from build123d import *

# Parameters (mm, degrees)
SKETCH_1_W          = 38
SKETCH_1_H          = 30
EXTRUDE_1_DEPTH     = 3
SKETCH_2_R          = 1.55
CUT_EXTRUDE_1_DEPTH = 10
SKETCH_3_W          = 22
SKETCH_3_H          = 22.358896132
CUT_EXTRUDE_2_DEPTH = 10
FILLET_1_R          = 7
FILLET_2_R          = 7
FILLET_3_R          = 3


with BuildPart() as part:
    # 草图1 → 凸台-拉伸1 (new body)
    with BuildSketch(Plane.XY):
        Rectangle(SKETCH_1_W, SKETCH_1_H)
    extrude(amount=EXTRUDE_1_DEPTH)

    # 草图2 → 切除-拉伸1 (cut)
    with BuildSketch(Plane.XY.offset(3)):
        with Locations((0, 12)):
            Circle(SKETCH_2_R)
        with Locations((-15, -12)):
            Circle(SKETCH_2_R)
        with Locations((15, -12)):
            Circle(SKETCH_2_R)
        with BuildLine():
            Line((6.963744532, 13.55), (13.036255468, 13.55))
            ThreePointArc((13.036255468, 13.55), (14.586255468, 12), (13.036255468, 10.45))
            Line((13.036255468, 10.45), (6.963744532, 10.45))
            ThreePointArc((6.963744532, 10.45), (5.413744532, 12), (6.963744532, 13.55))
        make_face()
        with BuildLine():
            Line((-6.963744532, 13.55), (-13.036255468, 13.55))
            ThreePointArc((-13.036255468, 13.55), (-14.586255468, 12), (-13.036255468, 10.45))
            Line((-13.036255468, 10.45), (-6.963744532, 10.45))
            ThreePointArc((-6.963744532, 10.45), (-5.413744532, 12), (-6.963744532, 13.55))
        make_face()
    extrude(amount=-CUT_EXTRUDE_1_DEPTH, mode=Mode.SUBTRACT)

    # 草图3 → 切除-拉伸2 (cut)
    with BuildSketch(Plane.XY.offset(3)):
        with Locations((0, -3.820551934)):
            Rectangle(SKETCH_3_W, SKETCH_3_H)
    extrude(amount=-CUT_EXTRUDE_2_DEPTH, mode=Mode.SUBTRACT)

    # 圆角1
    fillet_1_edges = [part.edges().sort_by_distance(p)[0] for p in [
        (-19, 15, 1.5),
        (19, 15, 1.5),
    ]]
    fillet(fillet_1_edges, radius=FILLET_1_R)

    # 圆角2
    fillet_2_edges = [part.edges().sort_by_distance(p)[0] for p in [
        (11, 7.358896132, 1.5),
        (-11, 7.358896132, 1.5),
    ]]
    fillet(fillet_2_edges, radius=FILLET_2_R)

    # 圆角3
    fillet_3_edges = [part.edges().sort_by_distance(p)[0] for p in [
        (11, -15, 1.5),
        (-11, -15, 1.5),
        (19, -15, 1.5),
        (-19, -15, 1.5),
    ]]
    fillet(fillet_3_edges, radius=FILLET_3_R)


solid = part.part
Geometry check sheet. Reference: the model listing, model coordinates, mm. A direction names the side the tool comes from. Round coordinates to 2 decimals unless told otherwise and drop trailing zeros. Order: outer loops, then holes, each group sorted by start corner. A loop starts at its lowest first (then second) coordinate and runs counter-clockwise, first axis right, second up. Notation, with made-up numbers: M -14,39.25 L 37,39.25 A29 cw 37,60.25 Z; hole C 55,77 d11. An arc over 180 degrees is marked long. Write each question's results on one line, items separated by ' | '. Start each with the question number.
1. Cross-section at B-B on z = 2.1. Record the boundary of the cut face in (x, y), plus the area to 3 significant figures.
2. Cross-section at A-A on x = 0. Record the boundary of the cut face in (y, z), plus the area to 3 significant figures.
3. Cross-section at C-C on y = -8.5. Record the boundary of the cut face in (x, z).
4. Go/stop test with flat-tipped pins: P1, Ø5, axis at x = -6, y = 0.5, coming from the -Z side; P2, Ø0.9, axis at x = -9.5, z = 2, coming from the -Y side. Record where each tip stops, or that it passes through.
5. Draft check along Y on faces 1 (the face through (-0.336, 10.487, 1.521)), 2 (the face through (0, 10, 3)), 3 (the face through (8.9, 5.36, 1.48)). Enter one of: pulls with the +Y half, pulls with the -Y half, needs draft (parallel to the pull), parting line crosses it, or undercut.
6. Set-up check for faces 4 (the face through (11, -6, 2)), 5 (the face through (10, 13.55, 2)), 6 (the face through (-15, -15, 1)): record each of +Z, -Z, +X, -X, +Y, -Y from which the full face is reachable in a straight line by a thin tool's end or side.
7. Cross-section at D-D on y = 12. Record the boundary of the cut face in (x, z), plus the area to 3 significant figures.
8. Material ranges on L1, parallel to X at y = 11.25, z = 2.55; L2, parallel to Y at x = 0, z = 1.75; L3, parallel to X at y = -11.25, z = 1.95, recorded low to high. Write a range as from..to.
Resolved:
1) outline: M -19,-12 A3 ccw -16,-15 L -14,-15 A3 ccw -11,-12 L -11,0.36 A7 cw -4,7.36 L 4,7.36 A7 cw 11,0.36 L 11,-12 A3 ccw 14,-15 L 16,-15 A3 ccw 19,-12 L 19,8 A7 ccw 12,15 L -12,15 A7 ccw -19,8 Z; hole C -15,-12 d3.1; hole M -13.04,10.45 L -6.96,10.45 A1.55 ccw -6.96,13.55 L -13.04,13.55 A1.55 ccw Z; hole C 0,12 d3.1; hole M 6.96,10.45 L 13.04,10.45 A1.55 ccw 13.04,13.55 L 6.96,13.55 A1.55 ccw Z; hole C 15,-12 d3.1 | area: 565 mm2
2) outline: M 7.36,0 L 10.45,0 L 10.45,3 L 7.36,3 Z; M 13.55,0 L 15,0 L 15,3 L 13.55,3 Z | area: 13.6 mm2
3) outline: M -19,0 L -11,0 L -11,3 L -19,3 Z; M 11,0 L 19,0 L 19,3 L 11,3 Z
4) P1: through | P2: y = 4.05
5) face 1: undercut | face 2: needs draft | face 3: pulls with the -Y half
6) face 4: +Z, -Z, -Y | face 5: +Z, -Z | face 6: +Z, -Z, +X, -X, -Y
7) outline: M -17.74,0 L -14.59,0 L -14.59,3 L -17.74,3 Z; M -5.41,0 L -1.55,0 L -1.55,3 L -5.41,3 Z; M 1.55,0 L 5.41,0 L 5.41,3 L 1.55,3 Z; M 14.59,0 L 17.74,0 L 17.74,3 L 14.59,3 Z | area: 42.1 mm2
8) L1: -18.2..-14.39, -5.61..-1.36, 1.36..5.61, 14.39..18.2 | L2: 7.36..10.45, 13.55..15 | L3: -19..-16.36, -13.64..-11, 11..13.64, 16.36..19
